Source: CAD feature listing. Evaluate the final solid. Frame: model axes, mm. Give positions to 0.01 mm unless a question says otherwise; leave off trailing zeros. Write each loop counter-clockwise with the first axis right and the second up, starting at its lowest first coordinate (ties: lowest second). Pieces come first, ordered by that corner, then holes. Notation, with made-up numbers: (-21.5, -17.75) -> (3.5, -17.75) arc R19 ccw to (3.5, 17.25) -> close; hole circle Ø5 at (5.5, 40.25). An arc over 180 degrees is marked (long way). Answer as a JSON object with one key per item and string values. Group by question number.
Item 1: Section query C-C on y = 1.75. Return the cut outline in (x, z) (3 decimals), plus the area to 3 significant figures.
Item 2: Pull-direction query (Y, two-part tool) for faces 1 (the face through (105.6, 5.8, 1.6)), 2 (the face through (112.39, 1.81, 1.61)), 3 (the face through (56, 12.7, 2)); classes: pulls with the +Y half, pulls with the -Y half, needs draft (parallel to the pull), parting line crosses it, or undercut.
Item 3: First-contact query: pin 1 Ø4.5 at (x, y) = (107.95, 6.35) entering from -Z. Flat tip, straight axial feed; report the tip coordinate or a pass-through.
Item 4: Section query A-A on z = 1.05. Give the number of separate pieces and of enclosed holes in the cut face, plus the area to 3 significant figures.
Item 5: Section query B-B on y = 7.75. Return the cut outline in (x, z) (3 decimals), plus the area to 3 significant figures.
Item 6: Ray query, probe 1 along X at (y, z) = (6.35, 1.6); probe 2 along Y at (x, z) = (6.35, 1.25); probe 3 along X at (y, z) = (8.25, 2.6). Return the intervals inside material, ascending. Write a range as from..to.
Solid Edge part; units mm, degrees
sketch "Sketch1" plane through (0, 0, 0) normal (0, 0, 1) x (1, 0, 0)
  line L0 (0, 0) -> (0, 12.7)
  line L1 (0, 12.7) -> (114.3, 12.7)
  line L2 (114.3, 12.7) -> (114.3, 0)
  line L3 (114.3, 0) -> (0, 0)
  dimension "D1" = 114.3
extrude "Protrusion1" add sketch "Sketch1" along normal blind 3.175
fillet "Round_1" radius 6.35 4 edges at (0, 12.7, 1.5875) (0, 0, 1.5875) (114.3, 0, 1.5875) (114.3, 12.7, 1.5875)
hole "Hole_1" at (6.35, 6.35, 0) direction (0, 0, 1) diameter 4.826 end through all
hole "Hole1" at (107.95, 6.35, 0) direction (0, 0, 1) diameter 4.826 end through all
properties part number "SR-06" material "Aluminum, 6061-T6"
Worked answers:
{
 "1": {"outline": "(1.972, 0) -> (112.328, 0) -> (112.328, 3.175) -> (1.972, 3.175) -> close", "area": "350 mm^2"},
 "2": {"face 1": "undercut", "face 2": "pulls with the -Y half", "face 3": "pulls with the +Y half"},
 "3": {"pin 1": "through"},
 "4": {"separate pieces": "1", "enclosed holes": "2", "area": "1,380 mm^2"},
 "5": {"outline": "(0.156, 0) -> (4.385, 0) -> (4.385, 3.175) -> (0.156, 3.175) -> close; (8.315, 0) -> (105.985, 0) -> (105.985, 3.175) -> (8.315, 3.175) -> close; (109.915, 0) -> (114.144, 0) -> (114.144, 3.175) -> (109.915, 3.175) -> close", "area": "337 mm^2"},
 "6": {"probe 1": "0..3.94, 8.76..105.54, 110.36..114.3", "probe 2": "0..3.94, 8.76..12.7", "probe 3": "0.29..4.86, 7.84..106.46, 109.44..114.01"}
}
